Build history of the part. All positions in model axes, mm. Give positions to 0.01 mm unless a question says otherwise; leave off trailing zeros. Write each loop counter-clockwise with the first axis right and the second up, starting at its lowest first coordinate (ties: lowest second). Pieces come first, ordered by that corner, then holes. Notation, with made-up numbers: (47, 69.25) -> (103, 69.25) arc R19 cw to (103, 86.25) -> close; hole circle Ø11 at (44, 78.5). An arc over 180 degrees is marked (long way). One line per question, with ' | ' between items. Start each with the question number.
(1) Pull direction X, two halves, no side cores. Call faces 1 (the flat face through (0, 0, -43)), 2 (the flat face through (0, 0, -8)): released by +X, released by -X, zero draft, split by the parting line, or undercut.
(2) Band-saw the part on B-B, the plane z = -38.5. Give the cut face in (x, y), and give its area (3 significant figures).
(3) Band-saw the part on A-A, the plane y = 1.4. Give the cut face in (x, z), and give its area (3 significant figures).
(4) Pin check, flat tips, straight feed: P1, Ø2, axis at x = -0.5, z = -28.5, coming from the +Y side; P2, Ø2, axis at y = -1.5, z = -28, coming from the -X side; P3, Ø0.6, axis at y = 1.5, z = 0.5, coming from the -X side; P4, Ø0.6, axis at x = 1.5, z = 0.5, coming from the +Y side. Stop position of each tip, or through.
(5) Drill centre lines: probe 1 along Y at (x, z) = (0, -3.75); probe 2 along X at (y, z) = (-0.1, -3); probe 3 along Z at (x, y) = (-1, 0.55). Where is each one in solid material? Low to high. Write a range as from..to.
from build123d import *

# Parameters (mm, degrees)
SKETCH_1_R          = 1.95
EXTRUDE_1_DEPTH     = 43
SKETCH_3_R          = 1
CUT_EXTRUDE_1_DEPTH = 8
EXTRUDE_START       = 0.5
EXTRUDE_3_DEPTH     = 0.5


with BuildPart() as part:
    # 草图1 → 凸台-拉伸1 (new body)
    with BuildSketch(Plane.XY):
        Circle(SKETCH_1_R)
    extrude(amount=-EXTRUDE_1_DEPTH)

    # 草图3 → 切除-拉伸1 (cut)
    with BuildSketch(Plane.XY):
        Circle(SKETCH_3_R)
    extrude(amount=-CUT_EXTRUDE_1_DEPTH, mode=Mode.SUBTRACT)

    # 草图4 → 凸台-拉伸3 (add)
    with BuildSketch(Plane.XY.offset(EXTRUDE_START)):
        with BuildLine():
            Line((-1.768728357, 0.2), (-1.939716474, 0.2))
            ThreePointArc((-1.939716474, 0.2), (-1.95, 0), (-1.939716474, -0.2))
            Line((-1.939716474, -0.2), (-1.768728357, -0.2))
            ThreePointArc((-1.768728357, -0.2), (-1.78, 0), (-1.768728357, 0.2))
        make_face()
        with BuildLine():
            ThreePointArc((1.95, 0), (1.947427422, 0.100132101), (1.939716474, 0.2))
            Line((1.939716474, 0.2), (1.768728357, 0.2))
            ThreePointArc((1.768728357, 0.2), (1.777179855, 0.100158687), (1.78, 0))
            ThreePointArc((1.78, 0), (1.777179855, -0.100158687), (1.768728357, -0.2))
            Line((1.768728357, -0.2), (1.939716474, -0.2))
            ThreePointArc((1.939716474, -0.2), (1.947427422, -0.100132101), (1.95, 0))
        make_face()
        with BuildLine():
            Line((0.2, -1.768728357), (0.2, -1.939716474))
            ThreePointArc((0.2, -1.939716474), (1.378858223, -1.378858223), (1.939716474, -0.2))
            Line((1.939716474, -0.2), (1.768728357, -0.2))
            ThreePointArc((1.768728357, -0.2), (1.258650071, -1.258650071), (0.2, -1.768728357))
        make_face()
        with BuildLine():
            Line((-0.2, -1.768728357), (-0.2, -1.939716474))
            ThreePointArc((-0.2, -1.939716474), (0, -1.95), (0.2, -1.939716474))
            Line((0.2, -1.939716474), (0.2, -1.768728357))
            ThreePointArc((0.2, -1.768728357), (0, -1.78), (-0.2, -1.768728357))
        make_face()
        with BuildLine():
            Line((-1.768728357, -0.2), (-1.939716474, -0.2))
            ThreePointArc((-1.939716474, -0.2), (-1.378858223, -1.378858223), (-0.2, -1.939716474))
            Line((-0.2, -1.939716474), (-0.2, -1.768728357))
            ThreePointArc((-0.2, -1.768728357), (-1.258650071, -1.258650071), (-1.768728357, -0.2))
        make_face()
        with BuildLine():
            ThreePointArc((-0.2, 1.939716474), (-1.378858223, 1.378858223), (-1.939716474, 0.2))
            Line((-1.939716474, 0.2), (-1.768728357, 0.2))
            ThreePointArc((-1.768728357, 0.2), (-1.258650071, 1.258650071), (-0.2, 1.768728357))
            Line((-0.2, 1.768728357), (-0.2, 1.939716474))
        make_face()
        with BuildLine():
            ThreePointArc((1.939716474, 0.2), (1.378858223, 1.378858223), (0.2, 1.939716474))
            Line((0.2, 1.939716474), (0.2, 1.768728357))
            ThreePointArc((0.2, 1.768728357), (1.258650071, 1.258650071), (1.768728357, 0.2))
            Line((1.768728357, 0.2), (1.939716474, 0.2))
        make_face()
        with BuildLine():
            ThreePointArc((0.2, 1.939716474), (0, 1.95), (-0.2, 1.939716474))
            Line((-0.2, 1.939716474), (-0.2, 1.768728357))
            ThreePointArc((-0.2, 1.768728357), (0, 1.78), (0.2, 1.768728357))
            Line((0.2, 1.768728357), (0.2, 1.939716474))
        make_face()
        with BuildLine():
            Line((-0.979795897, 0.2), (-1.768728357, 0.2))
            ThreePointArc((-1.768728357, 0.2), (-1.78, 0), (-1.768728357, -0.2))
            Line((-1.768728357, -0.2), (-0.979795897, -0.2))
            ThreePointArc((-0.979795897, -0.2), (-1, 0), (-0.979795897, 0.2))
        make_face()
        with BuildLine():
            ThreePointArc((1.78, 0), (1.777179855, 0.100158687), (1.768728357, 0.2))
            Line((1.768728357, 0.2), (0.979795897, 0.2))
            ThreePointArc((0.979795897, 0.2), (0.994936153, 0.100508962), (1, 0))
            ThreePointArc((1, 0), (0.994936153, -0.100508962), (0.979795897, -0.2))
            Line((0.979795897, -0.2), (1.768728357, -0.2))
            ThreePointArc((1.768728357, -0.2), (1.777179855, -0.100158687), (1.78, 0))
        make_face()
        with BuildLine():
            ThreePointArc((0.2, 1.768728357), (0, 1.78), (-0.2, 1.768728357))
            Line((-0.2, 1.768728357), (-0.2, 0.979795897))
            ThreePointArc((-0.2, 0.979795897), (0, 1), (0.2, 0.979795897))
            Line((0.2, 0.979795897), (0.2, 1.768728357))
        make_face()
        with BuildLine():
            Line((-0.2, -0.979795897), (-0.2, -1.768728357))
            ThreePointArc((-0.2, -1.768728357), (0, -1.78), (0.2, -1.768728357))
            Line((0.2, -1.768728357), (0.2, -0.979795897))
            ThreePointArc((0.2, -0.979795897), (0, -1), (-0.2, -0.979795897))
        make_face()
    extrude(amount=-EXTRUDE_3_DEPTH)


solid = part.part
Results:
1) face 1: zero draft | face 2: undercut
2) outline: circle Ø3.9 at (0, 0) | area: 11.9 mm²
3) outline: (-1.36, -43) -> (1.36, -43) -> (1.36, 0.5) -> (1.1, 0.5) -> (1.1, 0) -> (0.2, 0) -> (0.2, 0.5) -> (-0.2, 0.5) -> (-0.2, 0) -> (-1.1, 0) -> (-1.1, 0.5) -> (-1.36, 0.5) -> close | area: 117 mm²
4) P1: stops at y = 1.95 | P2: stops at x = -1.88 | P3: stops at x = -1.54 | P4: stops at y = 1.54
5) probe 1: y = -1.95..-1, 1..1.95 | probe 2: x = -1.95..-0.99, 0.99..1.95 | probe 3: z = -43..0
